The listing builds one solid part. Answer for the finished solid, in the listing's coordinates (mm). A direction names the side the tool comes from. Coordinates: 2 decimals unless noted, no trailing zeros. Order: outer loops, then holes, each group sorted by start corner. A loop starts at its lowest first (then second) coordinate and runs counter-clockwise, first axis right, second up. Notation, with made-up numbers: (79, 55.5) - (99, 55.5) arc R10 ccw to (99, 69.5) - close; hole circle Ø5 at (82.25, 24). An arc over 180 degrees is marked (long way). Use a Markdown table: item, result. Add a question column.
Item 1: For faces 5 (the flat face through (67.5, -1, -2)), 6 (the flat face through (-1, -47.425, -2)), 7 (the cylindrical face through (65.094, -45.144, -2.366)), determine the directions among +Z, -Z, +X, -X, +Y, -Y from which every point of the face is accessible in a straight line to the end or side of a thin tool.
Item 2: The mould has two halves that part along X. Classify faces 1 (the flat face through (-1, -48, 2.91)), 2 (the cylindrical face through (-76.951, -52.054, 1.435)), 3 (the cylindrical face through (65.22, 45.02, -2.37)), 4 (the flat face through (-14, 41, -2.09)): released by +X, released by -X, zero draft, split by the parting line, or undercut.
Item 3: Flat-ended cylindrical pins translate along their axes: P1, Ø2.5, axis at y = 15.5, z = -2.5, coming from the -X side; P2, Ø1.4, axis at y = 2.5, z = -3.5, coming from the +X side; P3, Ø4, axis at x = 21, z = -3, coming from the +Y side (3 decimals). Find the tip coordinate at first contact, or state that the pin passes through.
Item 4: The part is cut by section C-C, the plane z = -3.5. Give the vertices of the cut face in (x, y) (3 decimals).
Item 5: The part is cut by section A-A, the plane x = 0. Give the vertices of the cut face in (y, z) (3 decimals), then the cut area to 3 significant figures.
Item 6: The part is cut by section D-D, the plane x = 50. Give the vertices of the cut face in (y, z) (3 decimals).
Item 7: Find the intervals of material crossed by line 1 along Y through (x, z) = (0, -4.1) (3 decimals); line 2 along Y through (x, z) = (2, -0.5) (3 decimals); line 3 along X through (y, z) = (-16, 2) (3 decimals), in increasing order.
Item 8: The part is cut by section B-B, the plane y = 0. Give the vertices of the cut face in (x, z) (3 decimals), then the cut area to 3 significant figures.
from build123d import *

# Parameters (mm, degrees)
F0_R     = 1.55
F1_DEPTH = 2.91
F3_DEPTH = 4.8
F4_R     = 42.5
F5_DEPTH = 25
F4_R_2   = 45.5
F6_DEPTH = 5


with BuildPart() as f1:
    # F0 (on Top) → F1 (new body)
    with BuildSketch(Plane.XY):
        with BuildLine():
            Line((-70.875, -54.61), (70.875, -54.61))
            ThreePointArc((70.875, -54.61), (76.885408, -52.120408), (79.375, -46.11))
            Line((79.375, -46.11), (79.375, 46.11))
            ThreePointArc((79.375, 46.11), (76.885408, 52.120408), (70.875, 54.61))
            Line((70.875, 54.61), (-70.875, 54.61))
            ThreePointArc((-70.875, 54.61), (-76.885408, 52.120408), (-79.375, 46.11))
            Line((-79.375, 46.11), (-79.375, -46.11))
            ThreePointArc((-79.375, -46.11), (-76.885408, -52.120408), (-70.875, -54.61))
        make_face()
        with Locations((71.875, -45.11)):
            Circle(F0_R, mode=Mode.SUBTRACT)
        with Locations((-71.875, 45.11)):
            Circle(F0_R, mode=Mode.SUBTRACT)
    extrude(amount=F1_DEPTH)

    # F2 (on Top) → F3 (join)
    with BuildSketch(Plane.XY):
        with BuildLine():
            Line((-59.5, -47.425), (59.5, -47.425))
            ThreePointArc((59.5, -47.425), (65.156854, -45.081854), (67.5, -39.425))
            Line((67.5, -39.425), (67.5, 39.425))
            ThreePointArc((67.5, 39.425), (65.156854, 45.081854), (59.5, 47.425))
            Line((59.5, 47.425), (-59.5, 47.425))
            ThreePointArc((-59.5, 47.425), (-65.156854, 45.081854), (-67.5, 39.425))
            Line((-67.5, 39.425), (-67.5, -39.425))
            ThreePointArc((-67.5, -39.425), (-65.156854, -45.081854), (-59.5, -47.425))
        make_face()
    extrude(amount=-F3_DEPTH)

    # F4 (on face) → F5 (cut)
    with BuildSketch(Plane.XY.offset(2.91)):
        Circle(F4_R)
    extrude(amount=-F5_DEPTH, mode=Mode.SUBTRACT)

    # F4 (on face) → F6 (cut)
    with BuildSketch(Plane.XY.offset(2.91)):
        Circle(F4_R_2)
        Circle(F4_R, mode=Mode.SUBTRACT)
    extrude(amount=-F6_DEPTH, mode=Mode.SUBTRACT)


solid = f1.part
Solution:
| question | item | result |
|---|---|---|
| 1 | face 5 | -Z, +X, +Y, -Y |
| 1 | face 6 | -Z, +X, -X, -Y |
| 1 | face 7 | -Z, +X, -Y |
| 2 | face 1 | zero draft |
| 2 | face 2 | released by -X |
| 2 | face 3 | released by +X |
| 2 | face 4 | undercut |
| 3 | P1 | stops at x = -67.5 |
| 3 | P2 | stops at x = 67.5 |
| 3 | P3 | stops at y = 47.425 |
| 4 | outline | (-67.5, -39.425) arc R8 ccw to (-59.5, -47.425) - (59.5, -47.425) arc R8 ccw to (67.5, -39.425) - (67.5, 39.425) arc R8 ccw to (59.5, 47.425) - (-59.5, 47.425) arc R8 ccw to (-67.5, 39.425) - close; hole circle Ø85 at (0, 0) |
| 5 | outline | (-54.61, 0) - (-47.425, 0) - (-47.425, -4.8) - (-42.5, -4.8) - (-42.5, -2.09) - (-45.5, -2.09) - (-45.5, 2.91) - (-54.61, 2.91) - close; (42.5, -4.8) - (47.425, -4.8) - (47.425, 0) - (54.61, 0) - (54.61, 2.91) - (45.5, 2.91) - (45.5, -2.09) - (42.5, -2.09) - close |
| 5 | area | 87.8 mm2 |
| 6 | outline | (-54.61, 0) - (-47.425, 0) - (-47.425, -4.8) - (47.425, -4.8) - (47.425, 0) - (54.61, 0) - (54.61, 2.91) - (-54.61, 2.91) - close |
| 7 | line 1 | y = -47.425 to -42.5, 42.5 to 47.425 |
| 7 | line 2 | y = -47.425 to -45.456, 45.456 to 47.425 |
| 7 | line 3 | x = -79.375 to -42.594, 42.594 to 79.375 |
| 8 | outline | (-79.375, 0) - (-67.5, 0) - (-67.5, -4.8) - (-42.5, -4.8) - (-42.5, -2.09) - (-45.5, -2.09) - (-45.5, 2.91) - (-79.375, 2.91) - close; (42.5, -4.8) - (67.5, -4.8) - (67.5, 0) - (79.375, 0) - (79.375, 2.91) - (45.5, 2.91) - (45.5, -2.09) - (42.5, -2.09) - close |
| 8 | area | 425 mm2 |
